Input: dimensioned drawing with shaded views. Units: mm. Origin: part minimum x, y, z. Round coordinates to 2 decimals unless told otherwise and drop trailing zeros. Loops run counter-clockwise (first coordinate to the right, second up) from the corner with the lowest first, then second, coordinate; pieces in that order, holes last. Notation, with made-up numbers: (-6, 10.5) - (8, 10.5) arc R16 cw to (8, 41.5) - close; hole circle Ø8 at (8.25, 64). An arc over 180 degrees is marked (long way). Answer as CSV lines item,"result".
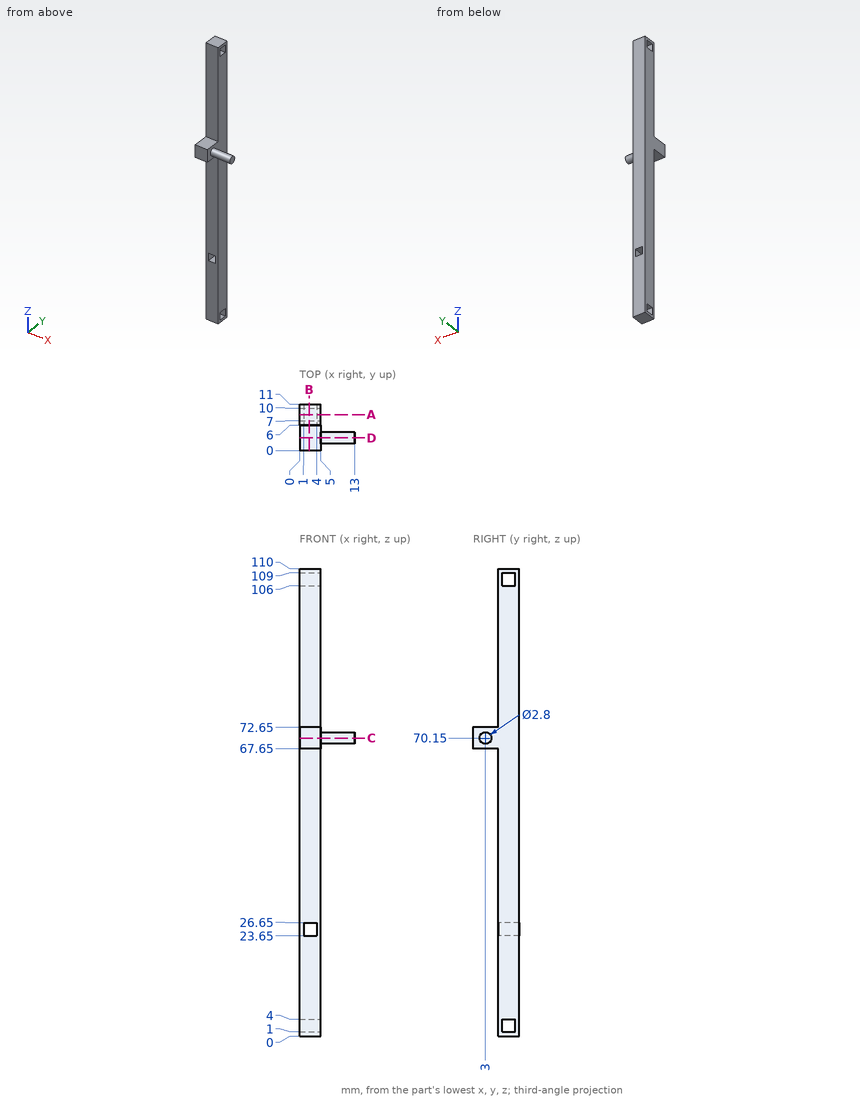
(1) Pin query (flat end, axial travel): P1, Ø2.5, axis at x = 3.5, z = 83.5, coming from the -Y side; P2, Ø1.5, axis at y = 7.5, z = 25, coming from the +X side; P3, Ø2, axis at x = 3.5, y = 1.5, coming from the -Z side. Return the tip coordinate at first contact, or that it passes through.
Findings below:
P1,"y = 6"
P2,"x = 5"
P3,"z = 67.65"
(2) Section A-A (y = 8.5). Output: boundary loops of the cut face in (x, z), and give its area (3 significant figures).
Findings below:
outline,"(0, 0) - (5, 0) - (5, 1) - (0, 1) - close; (0, 4) - (5, 4) - (5, 106) - (0, 106) - close; (0, 109) - (5, 109) - (5, 110) - (0, 110) - close; hole (1, 23.65) - (4, 23.65) - (4, 26.65) - (1, 26.65) - close"
area,"511 mm2"
(3) Section D-D (y = 3). Output: boundary loops of the cut face in (x, z), and give its area (3 significant figures).
Findings below:
outline,"(0, 67.65) - (5, 67.65) - (5, 68.75) - (13, 68.75) - (13, 71.55) - (5, 71.55) - (5, 72.65) - (0, 72.65) - close"
area,"47.4 mm2"
(4) Section C-C (z = 70.15). Output: boundary loops of the cut face in (x, y), and give its area (3 significant figures).
Findings below:
outline,"(0, 0) - (5, 0) - (5, 1.6) - (13, 1.6) - (13, 4.4) - (5, 4.4) - (5, 11) - (0, 11) - close"
area,"77.4 mm2"
(5) Section B-B (x = 2.25). Output: boundary loops of the cut face in (y, z), and give its area (3 significant figures).
Findings below:
outline,"(0, 67.65) - (6, 67.65) - (6, 26.65) - (11, 26.65) - (11, 110) - (6, 110) - (6, 72.65) - (0, 72.65) - close; (6, 0) - (11, 0) - (11, 23.65) - (6, 23.65) - close; hole (7, 1) - (10, 1) - (10, 4) - (7, 4) - close; hole (7, 106) - (10, 106) - (10, 109) - (7, 109) - close"
area,"547 mm2"
(6) Material intervals for line 1 along Z through (x, y) = (4.25, 8.75); line 2 along Z through (x, y) = (4, 5.75); line 3 along Y through (x, z) = (4.25, 79.5), sorted ascending.
Findings below:
line 1,"0 to 1, 4 to 106, 109 to 110"
line 2,"67.65 to 72.65"
line 3,"6 to 11"
